```python
from build123d import *

# Parameters (mm, degrees)
SKETCH_1_R      = 1.5
EXTRUDE_1_DEPTH = 1.5


with BuildPart() as part:
    # 草图1 → 凸台-拉伸1 (new body)
    with BuildSketch(Plane.XY):
        with BuildLine():
            Line((-43.535533906, 21.464466094), (-30, 7.928932188))
            Line((-30, 7.928932188), (-30, -7.928932188))
            Line((-30, -7.928932188), (-43.535533906, -21.464466094))
            ThreePointArc((-43.535533906, -21.464466094), (-43.535533906, -28.535533906), (-36.464466094, -28.535533906))
            Line((-36.464466094, -28.535533906), (-22.928933621, -15.000001433))
            Line((-22.928933621, -15.000001433), (22.928933621, -15.000001433))
            Line((22.928933621, -15.000001433), (36.464466094, -28.535533906))
            ThreePointArc((36.464466094, -28.535533906), (43.535533906, -28.535533906), (43.535533906, -21.464466094))
            Line((43.535533906, -21.464466094), (30, -7.928932188))
            Line((30, -7.928932188), (30, 7.928932188))
            Line((30, 7.928932188), (43.535533906, 21.464466094))
            ThreePointArc((43.535533906, 21.464466094), (43.535533906, 28.535533906), (36.464466094, 28.535533906))
            Line((36.464466094, 28.535533906), (22.928933621, 15.000001433))
            Line((22.928933621, 15.000001433), (-22.928933621, 15.000001433))
            Line((-22.928933621, 15.000001433), (-36.464466094, 28.535533906))
            ThreePointArc((-36.464466094, 28.535533906), (-43.535533906, 28.535533906), (-43.535533906, 21.464466094))
        make_face()
        with Locations((-40, 25)):
            Circle(SKETCH_1_R, mode=Mode.SUBTRACT)
        with Locations((40, 25)):
            Circle(SKETCH_1_R, mode=Mode.SUBTRACT)
        with Locations((40, -25)):
            Circle(SKETCH_1_R, mode=Mode.SUBTRACT)
        with Locations((-40, -25)):
            Circle(SKETCH_1_R, mode=Mode.SUBTRACT)
    extrude(amount=EXTRUDE_1_DEPTH)


solid = part.part
```
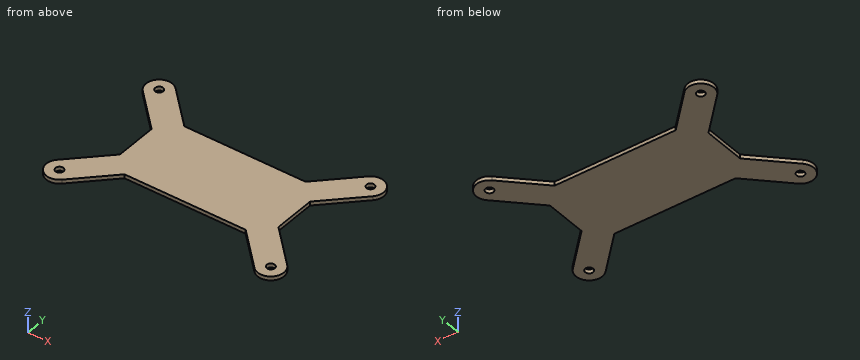
Build history of the part. All positions in model axes, mm. Give positions to 0.01 mm unless a question says otherwise; leave off trailing zeros. Loops run counter-clockwise (first coordinate to the right, second up) from the corner with the lowest first, then second, coordinate; pieces in that order, holes last.
Item 1: Slice it at D-D, the plane x = -6. List the corners of the cut face in (y, z).
Answers follow:
outline: (-15, 0) - (15, 0) - (15, 1.5) - (-15, 1.5) - close
Item 2: Slice it at A-A, the plane z = 0.5. List the corners of the cut face in (x, y).
Answers follow:
outline: (-43.54, -21.46) arc R5 ccw to (-36.46, -28.54) - (-22.93, -15) - (22.93, -15) - (36.46, -28.54) arc R5 ccw to (43.54, -21.46) - (30, -7.93) - (30, 7.93) - (43.54, 21.46) arc R5 ccw to (36.46, 28.54) - (22.93, 15) - (-22.93, 15) - (-36.46, 28.54) arc R5 ccw to (-43.54, 21.46) - (-30, 7.93) - (-30, -7.93) - close; hole circle Ø3 at (-40, -25); hole circle Ø3 at (-40, 25); hole circle Ø3 at (40, -25); hole circle Ø3 at (40, 25)
Item 3: Slice it at C-C, the plane x = 40. List the corners of the cut face in (y, z).
Answers follow:
outline: (-30, 0) - (-26.5, 0) - (-26.5, 1.5) - (-30, 1.5) - close; (-23.5, 0) - (-17.93, 0) - (-17.93, 1.5) - (-23.5, 1.5) - close; (17.93, 0) - (23.5, 0) - (23.5, 1.5) - (17.93, 1.5) - close; (26.5, 0) - (30, 0) - (30, 1.5) - (26.5, 1.5) - close
Item 4: Flat gauge pins, fed straight in: pin 1 (3 mm diameter, centred on x = 10, y = 4, fed in from -Z); pin 2 (0.8 mm diameter, centred on y = 1.5, z = 0.5, fed in from +X); pin 3 (0.8 mm diameter, centred on x = -5.5, z = 1, fed in from -Y). Where does each tip first touch, or does it go through?
Answers follow:
pin 1: stops at z = 0
pin 2: stops at x = 30
pin 3: stops at y = -15
Item 5: Slice it at B-B, the plane y = -25. List the corners of the cut face in (x, z).
Answers follow:
outline: (-45, 0) - (-41.5, 0) - (-41.5, 1.5) - (-45, 1.5) - close; (-38.5, 0) - (-32.93, 0) - (-32.93, 1.5) - (-38.5, 1.5) - close; (32.93, 0) - (38.5, 0) - (38.5, 1.5) - (32.93, 1.5) - close; (41.5, 0) - (45, 0) - (45, 1.5) - (41.5, 1.5) - close
Item 6: Drill centre lines: line 1 (Y direction, x = -40, z = 0.3); line 2 (X direction, y = 25.5, z = 1.2); line 3 (Y direction, x = -9, z = 0.4). Where is each one in solid material? Low to high.
Answers follow:
line 1: y = -30 to -26.5, -23.5 to -17.93, 17.93 to 23.5, 26.5 to 30
line 2: x = -44.97 to -41.41, -38.59 to -33.43, 33.43 to 38.59, 41.41 to 44.97
line 3: y = -15 to 15
